from build123d import *

# Parameters (mm, degrees)
MODEL_R                 = 1.5
MODEL_W                 = 3
MODEL_H                 = 3
SALIENTE_EXTRUIR1_DEPTH = 3


with BuildPart() as part:
    # Model → Saliente-Extruir1 (new body)
    with BuildSketch(Plane.XY):
        with BuildLine():
            Line((11.668043303, 286.574114522), (11.668043303, 280.829551876))
            ThreePointArc((11.668043303, 280.829551876), (11.781638042, 280.366641826), (12.096614731, 280.008900069))
            ThreePointArc((12.096614731, 280.008900069), (12.790231402, 279.612356159), (13.543043303, 279.344726935))
            ThreePointArc((13.543043303, 279.344726935), (15.173719263, 278.545183038), (16.355543303, 277.166173803))
            ThreePointArc((16.355543303, 277.166173803), (20.67525751, 272.472044196), (26.668043303, 270.285425334))
            Line((26.668043303, 270.285425334), (26.668043303, 276.576833199))
            Line((26.668043303, 276.576833199), (25.668043303, 276.576833199))
            ThreePointArc((25.668043303, 276.576833199), (25.137713217, 276.796503113), (24.918043303, 277.326833199))
            Line((24.918043303, 277.326833199), (24.918043303, 279.076833199))
            ThreePointArc((24.918043303, 279.076833199), (25.137713217, 279.607163285), (25.668043303, 279.826833199))
            Line((25.668043303, 279.826833199), (26.668043303, 279.826833199))
            Line((26.668043303, 279.826833199), (26.668043303, 287.576833199))
            Line((26.668043303, 287.576833199), (25.668043303, 287.576833199))
            ThreePointArc((25.668043303, 287.576833199), (25.137713217, 287.796503113), (24.918043303, 288.326833199))
            Line((24.918043303, 288.326833199), (24.918043303, 290.076833199))
            ThreePointArc((24.918043303, 290.076833199), (25.137713217, 290.607163285), (25.668043303, 290.826833199))
            Line((25.668043303, 290.826833199), (26.668043303, 290.826833199))
            Line((26.668043303, 290.826833199), (26.668043303, 297.118241064))
            ThreePointArc((26.668043303, 297.118241064), (20.67525751, 294.931622203), (16.355543303, 290.237492596))
            ThreePointArc((16.355543303, 290.237492596), (15.173719263, 288.858483361), (13.543043303, 288.058939464))
            ThreePointArc((13.543043303, 288.058939464), (12.790231402, 287.79131024), (12.096614731, 287.394766329))
            ThreePointArc((12.096614731, 287.394766329), (11.781638042, 287.037024572), (11.668043303, 286.574114522))
        make_face()
        with Locations((14.668043303, 283.701833199)):
            Circle(MODEL_R, mode=Mode.SUBTRACT)
        with Locations((19.168043303, 288.201833199)):
            Rectangle(MODEL_W, MODEL_H, mode=Mode.SUBTRACT)
        with Locations((19.168043303, 279.201833199)):
            Rectangle(MODEL_W, MODEL_H, mode=Mode.SUBTRACT)
    extrude(amount=SALIENTE_EXTRUIR1_DEPTH)


solid = part.part
Design review of the part built by this model. Coordinates are the model's own, in mm. A direction names the side the tool comes from. Give positions to 0.01 mm unless a question says otherwise; leave off trailing zeros. Loops run counter-clockwise (first coordinate to the right, second up) from the corner with the lowest first, then second, coordinate; pieces in that order, holes last. Notation, with made-up numbers: (15.5, 22.25) - (74.5, 22.25) arc R33 cw to (74.5, 57.25) - close; hole circle Ø1 at (1, 26). An arc over 180 degrees is marked (long way). Use CSV: the item, a comma, the result in double quotes. Start each with the question number.
1. Draft analysis for pull direction Y (two halves, no side actions). For faces 4 (the flat face through (11.668, 284, 1)), 5 (the cylindrical face through (11.785, 287.043, 1.479)), 6 (the cylindrical face through (20.6, 272.522, 1.479)), 7 (the flat face through (20.668, 288, 1)), state which applies: released by +Y, released by -Y, zero draft, split by the parting line, or undercut.
2. Insertion check: P1, Ø0.9, axis at y = 289, z = 1, coming from the +X side; P2, Ø1.5, axis at y = 289, z = 1.5, coming from the -X side; P3, Ø0.8, axis at x = 26, z = 2, coming from the -Y side. Each pin has a flat end and moves straight along its axis. Give the tip position at first contact, or say it passes through.
3. Add section D-D (y = 274.75). State the section outline as (x, z) points.
4. Add section B-B (z = 1.75). Count the separate pieces of the cut face and the enclosed holes in it, plus the area to 3 significant figures.
5. Machinability: for faces 1 (the flat face through (21, 284, 0)), 2 (the flat face through (24.918, 289, 1)), 3 (the flat face through (17.668, 288, 1)), which of the approach directions +Z, -Z, +X, -X, +Y, -Y give a long, thin tool a straight path to every point of the face, cutting with its end or side? Answer none if there is none.
6. Add section C-C (x = 18.75). State the section outline as (y, z) points.
7. Wall thickness on L1, parallel to Y at x = 18.5, z = 0.55; L2, parallel to Y at x = 19, z = 2.4; L3, parallel to X at y = 288.25, z = 0.7: over which ranges is each line inside the solid? List them lowest first.
8. Add section A-A (y = 288.75). State the section outline as (x, z) points, plus the area to 3 significant figures.
Results found:
1,face 4,"zero draft"
1,face 5,"released by +Y"
1,face 6,"released by -Y"
1,face 7,"undercut"
2,P1,"stops at x = 24.92"
2,P2,"stops at x = 14.12"
2,P3,"stops at y = 270.32"
3,outline,"(18.06, 0) - (26.67, 0) - (26.67, 3) - (18.06, 3) - close"
4,separate pieces,"1"
4,enclosed holes,"3"
4,area,"239 mm²"
5,face 1,"-Z, +X, -X, +Y, -Y"
5,face 2,"+Z, -Z, +X"
5,face 3,"+Z, -Z"
6,outline,"(274.03, 0) - (277.7, 0) - (277.7, 3) - (274.03, 3) - close; (280.7, 0) - (286.7, 0) - (286.7, 3) - (280.7, 3) - close; (289.7, 0) - (293.37, 0) - (293.37, 3) - (289.7, 3) - close"
7,L1,"y = 274.28 to 277.7, 280.7 to 286.7, 289.7 to 293.12"
7,L2,"y = 273.79 to 277.7, 280.7 to 286.7, 289.7 to 293.61"
7,L3,"x = 14.12 to 17.67, 20.67 to 24.92"
8,outline,"(15.03, 0) - (17.67, 0) - (17.67, 3) - (15.03, 3) - close; (20.67, 0) - (24.92, 0) - (24.92, 3) - (20.67, 3) - close"
8,area,"20.7 mm²"
